from build123d import *

# Parameters (mm, degrees)
SKETCH1_R                = 4
BOSS_EXTRUDE1_DEPTH      = 16
CUT_EXTRUDE2_DEPTH       = 243.712011885
FILLET2_R                = 50
FILLET3_R                = 5
BOSS_EXTRUDE2_DEPTH      = 16
LPATTERN1_COUNT          = 58
LPATTERN1_PITCH          = 5
SKETCH6_R                = 5.25
CUT_EXTRUDE4_DEPTH       = 3.2
BOSS_EXTRUDE3_START      = -11.8
SKETCH8_R                = 4
SKETCH8_R_2              = 2
BOSS_EXTRUDE3_DEPTH      = 11.8
SKETCH9_R                = 5
CUT_EXTRUDE7_DEPTH       = 9.8
BOSS_EXTRUDE4_DEPTH      = 16
CUT_EXTRUDE8_DEPTH       = 330.19878797
CUT_EXTRUDE8_DEPTH_BACK  = 330.19878797
SKETCH10_R               = 3.15
CUT_EXTRUDE9_DEPTH       = 230.693221824
CUT_EXTRUDE10_DEPTH      = 230.693221824
CUT_EXTRUDE13_DEPTH      = 228.62792195
FILLET6_R                = 15
FILLET7_R                = 2
SKETCH18_R               = 11
CUT_EXTRUDE14_DEPTH      = 180
CUT_EXTRUDE15_DEPTH      = 211.145198264
CUT_EXTRUDE15_DEPTH_BACK = 211.145198264
BOSS_EXTRUDE5_REACH      = 203.817
FILLET8_R                = 1
FILLET9_R                = 3
CUT_EXTRUDE16_DEPTH      = 239.866298177
CUT_EXTRUDE16_DEPTH_BACK = 239.866298177
SKETCH21_R               = 3.15


with BuildPart() as part:
    # Sketch1 → Boss-Extrude1 (new body)
    with BuildSketch(Plane(origin=(0, 0, 0), x_dir=(1, 0, 0), z_dir=(0, 1, 0))):
        Polygon((0, 0), (-70, 135), (-70, -15), (-70, -215), (111.481481481, -215), align=None)
        with Locations(Location((-5, -5, 0), (0, 0, 270))):
            Circle(SKETCH1_R, mode=Mode.SUBTRACT)
    extrude(amount=BOSS_EXTRUDE1_DEPTH)

    # Sketch3 → Cut-Extrude2 (cut, through all)
    with BuildSketch(Plane(origin=(0, 16, 0), x_dir=(1, 0, 0), z_dir=(0, 1, 0))):
        Polygon((-52.442610269, 88.104828667), (-69.618224346, 82.719823463), (14.148523277, -184.456395525), (31.324137355, -179.07139032), align=None)
    extrude(amount=-CUT_EXTRUDE2_DEPTH, mode=Mode.SUBTRACT)

    # Fillet2
    fillet2_edges = [part.edges().sort_by_distance(p)[0] for p in [
        (111.481481481, 8, 215),
        (-70, 8, 215),
    ]]
    fillet(fillet2_edges, radius=FILLET2_R)

    # Fillet3
    fillet3_edges = [part.edges().sort_by_distance(p)[0] for p in [
        (-70, 8, -135),
    ]]
    fillet(fillet3_edges, radius=FILLET3_R)

    # Sketch4 → Boss-Extrude2 (add)
    with BuildSketch(Plane(origin=(0, 16, 0), x_dir=(1, 0, 0), z_dir=(0, 1, 0))):
        Polygon((-60.561227343, 116.796652732), (-54.510866943, 115.99017648), (-58.9496396, 113.688590657), align=None)
    boss_extrude2 = extrude(amount=-BOSS_EXTRUDE2_DEPTH)

    # LPattern1: Boss-Extrude2 ×58
    with Locations(*[Vector(0.46031716445500054, 0, 0.8877545314489294) * (i * LPATTERN1_PITCH) for i in range(1, LPATTERN1_COUNT)]):
        add(boss_extrude2)

    # Sketch6 → Cut-Extrude4 (cut)
    with BuildSketch(Plane.XZ):
        with Locations(Location((-5, 5, 0), (0, 0, 270))):
            Circle(SKETCH6_R)
    extrude(amount=-CUT_EXTRUDE4_DEPTH, mode=Mode.SUBTRACT)

    # Sketch8 → Boss-Extrude3 (add)
    with BuildSketch(Plane(origin=(0, 16, 0), x_dir=(1, 0, 0), z_dir=(0, 1, 0)).offset(BOSS_EXTRUDE3_START)):
        with Locations(Location((-5, -5, 0), (0, 0, 90))):
            Circle(SKETCH8_R)
        with Locations(Location((-5, -5, 0), (0, 0, 270))):
            Circle(SKETCH8_R_2, mode=Mode.SUBTRACT)
    extrude(amount=BOSS_EXTRUDE3_DEPTH)

    # Sketch9 → Cut-Extrude7 (cut)
    with BuildSketch(Plane(origin=(0, 16, 0), x_dir=(1, 0, 0), z_dir=(0, 1, 0))):
        with Locations(Location((-5, -5, 0), (0, 0, 270))):
            Circle(SKETCH9_R)
    extrude(amount=-CUT_EXTRUDE7_DEPTH, mode=Mode.SUBTRACT)

    # Sketch12 → Boss-Extrude4 (add)
    with BuildSketch(Plane(origin=(0, 16, 0), x_dir=(1, 0, 0), z_dir=(0, 1, 0))):
        with BuildLine():
            Line((-70, 114.49506691), (-70, 54.49506691))
            ThreePointArc((-70, 54.49506691), (-73.030615433, 84.49506691), (-70, 114.49506691))
        make_face()
    extrude(amount=-BOSS_EXTRUDE4_DEPTH)

    # Sketch10 → Cut-Extrude8 (cut, two sides: drawn at the far end of the back side and taken through both)
    with BuildSketch(Plane(origin=(-29.844534263, 0, -95.189917814), x_dir=(0.954200782099043, 0, -0.29916695579822083), z_dir=(0.29916695579822083, 0, 0.954200782099043)).offset(-CUT_EXTRUDE8_DEPTH_BACK)):
        with Locations(Location((-32.68272635, 8, 0), (0, 0, 272.580314011))):
            Circle(SKETCH10_R)
    extrude(amount=CUT_EXTRUDE8_DEPTH + CUT_EXTRUDE8_DEPTH_BACK, mode=Mode.SUBTRACT)

    # Sketch13 → Cut-Extrude9 (cut, through all)
    with BuildSketch(Plane(origin=(0, 16, 0), x_dir=(1, 0, 0), z_dir=(0, 1, 0))):
        Polygon((-74.389228257, 81.223988684), (30.319206273, -252.746285051), (-65.100871937, -282.662980631), (-169.809306467, 51.307293104), align=None)
    extrude(amount=-CUT_EXTRUDE9_DEPTH, mode=Mode.SUBTRACT)

    # Sketch15 → Cut-Extrude10 (cut, through all)
    with BuildSketch(Plane(origin=(0, 16, 0), x_dir=(1, 0, 0), z_dir=(0, 1, 0))):
        Polygon((91.161899767, -18.950897803), (-4.258178443, -48.867593383), (70.533560507, -287.417788908), (165.953638717, -257.501093328), align=None)
    extrude(amount=-CUT_EXTRUDE10_DEPTH, mode=Mode.SUBTRACT)

    # Sketch16 → Cut-Extrude13 (cut, through all)
    with BuildSketch(Plane(origin=(0, 16, 0), x_dir=(1, 0, 0), z_dir=(0, 1, 0))):
        with BuildLine():
            Line((10.873354146, -190.723234214), (40.790049725, -286.143312424))
            Line((40.790049725, -286.143312424), (67.507671624, -277.766637662))
            Line((67.507671624, -277.766637662), (37.590976044, -182.346559452))
            ThreePointArc((37.590976044, -182.346559452), (27.10860607, -195.709380094), (10.873354146, -190.723234214))
        make_face()
    extrude(amount=-CUT_EXTRUDE13_DEPTH, mode=Mode.SUBTRACT)

    # Fillet6
    fillet6_edges = [part.edges().sort_by_distance(p)[0] for p in [
        (-4.258178443, 8, 48.867593383),
    ]]
    fillet(fillet6_edges, radius=FILLET6_R)

    # Fillet7
    fillet7_edges = [part.edges().sort_by_distance(p)[0] for p in [
        (-52.442610269, 8, -88.104828667),
        (31.324137355, 8, 179.07139032),
        (14.148523277, 8, 184.456395525),
        (-69.618224346, 8, -82.719823463),
    ]]
    fillet(fillet7_edges, radius=FILLET7_R)

    # Sketch18 → Cut-Extrude14 (cut)
    with BuildSketch(Plane(origin=(53.92221336, 0, 171.986301173), x_dir=(-0.9542007820990451, 0, 0.2991669557982141), z_dir=(-0.2991669557982141, 0, -0.9542007820990451))):
        with Locations((32.68272635, 8)):
            Circle(SKETCH18_R)
    extrude(amount=CUT_EXTRUDE14_DEPTH, mode=Mode.SUBTRACT)

    # Sketch19 → Cut-Extrude15 (cut, two sides: drawn at the far end of the back side and taken through both)
    with BuildSketch(Plane(origin=(0, 16, 0), x_dir=(1, 0, 0), z_dir=(0, 1, 0)).offset(-CUT_EXTRUDE15_DEPTH_BACK)):
        Polygon((-23.735854186, 45.776290217), (-43.616849953, -16.925311817), (-182.188010341, 92.887453174), (-34.776254673, 144.843881828), (-3.278660629, 45.963592539), align=None)
    extrude(amount=CUT_EXTRUDE15_DEPTH + CUT_EXTRUDE15_DEPTH_BACK, mode=Mode.SUBTRACT)

    # Boss-Extrude5: up to this face of the body (flat: up to its plane)
    boss_extrude5_end = Plane(part.part.faces().sort_by_distance((-3.292295487, 0, 60.867970257))[0])
    # Sketch20 → Boss-Extrude5 (add, up to the picked face)
    with BuildSketch(Plane(origin=(0, 16, 0), x_dir=(1, 0, 0), z_dir=(0, 1, 0)), mode=Mode.PRIVATE) as boss_extrude5_sk1:
        Polygon((-31.497089872, 21.298546901), (-40.982119501, -8.615777313), (-36.494615164, -22.928789044), (-19.319001086, -17.54378384), align=None)
    boss_extrude5_tool1 = split(extrude(boss_extrude5_sk1.sketch, amount=-BOSS_EXTRUDE5_REACH, mode=Mode.PRIVATE), bisect_by=boss_extrude5_end, keep=Keep.BOTH, mode=Mode.PRIVATE)
    add(boss_extrude5_tool1.solids().sort_by(Axis((-31.047961, 16, 5.590001), (0, -1, 0)))[0])

    # Fillet8
    fillet8_edges = [part.edges().sort_by_distance(p)[0] for p in [
        (-36.494615164, 15.16227766, 22.928789044),
        (-36.494615164, 0.83772234, 22.928789044),
        (-19.319001086, 0.83772234, 17.54378384),
        (-19.319001086, 15.16227766, 17.54378384),
    ]]
    fillet(fillet8_edges, radius=FILLET8_R)

    # Fillet9
    fillet9_edges = [part.edges().sort_by_distance(p)[0] for p in [
        (-23.735854186, 8, -45.776290217),
    ]]
    fillet(fillet9_edges, radius=FILLET9_R)

    # Sketch21 → Cut-Extrude16 (cut, two sides: drawn at the far end of the back side and taken through both)
    with BuildSketch(Plane(origin=(53.92221336, 0, 171.986301173), x_dir=(-0.9542007820990451, 0, 0.2991669557982141), z_dir=(-0.2991669557982141, 0, -0.9542007820990451)).offset(-CUT_EXTRUDE16_DEPTH_BACK)):
        with Locations(Location((32.68272635, 8, 0), (0, 0, 180))):
            Circle(SKETCH21_R)
    extrude(amount=CUT_EXTRUDE16_DEPTH + CUT_EXTRUDE16_DEPTH_BACK, mode=Mode.SUBTRACT)


solid = part.part
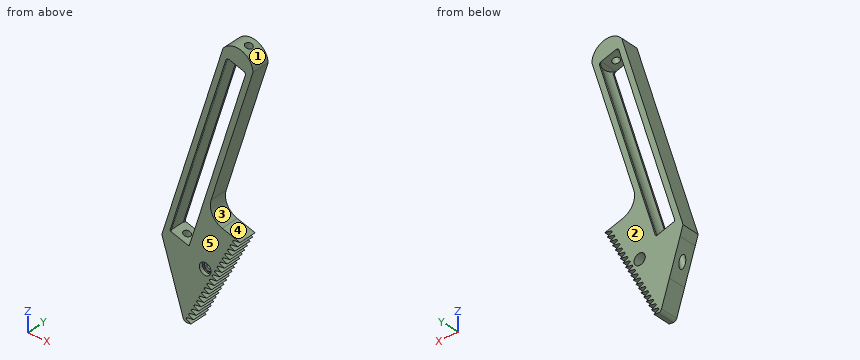
Build history of the part. All positions in model axes, mm. Face numbers are marked on the shaded views. A direction names the side the tool comes from. Coordinates: 2 decimals unless noted, no trailing zeros. Write each question's results on one line, items separated by ' | '. Start each with the question number.
Item 1: Mould opens along Z. For the marked faces 1, 2 and 3 say: released by +Z, released by -Z, zero draft, split by the parting line, or undercut.
Item 2: Flat gauge pins, fed straight in: pin 1 (2 mm diameter, centred on x = 16.5, y = 8, fed in from +Z); pin 2 (3 mm diameter, centred on x = -6.5, z = 3.5, fed in from -Y); pin 3 (4 mm diameter, centred on x = -6, z = 3, fed in from -Y). Where does each tip first touch, or does it go through?
Item 3: Tool access for the marked faces 4 and 5: list every direction of +Z, -Z, +X, -X, +Y, -Y with a clear straight run to the whole face (end or side of a thin tool).
Item 4: Wall check: probe 1 along X at (y, z) = (5.5, 5); probe 2 along X at (y, z) = (9.25, 5); probe 3 along X at (y, z) = (4.05, 5). Give the ranges that are in metal, low to high. Write a range as [from, to].
Numbers:
1) face 1: released by +Z | face 2: zero draft | face 3: undercut
2) pin 1: z = 195.5 | pin 2: y = 4.2 | pin 3: y = 3.2
3) face 4: +X, +Y, -Y | face 5: +Z, -Z, +X, -X, -Y
4) probe 1: [-39.84, -34.69], [-30.68, -7], [-3, 5.43] | probe 2: [-39.84, -35.71], [-29.65, -10], [0, 5.43] | probe 3: [-39.84, -9], [-1, 5.43]
